For this review, take the finished solid that the model builds, in its own axes (mm). Face numbers are marked on the shaded views. Round coordinates to 2 decimals unless told otherwise and drop trailing zeros. Loops run counter-clockwise (first coordinate to the right, second up) from the corner with the lowest first, then second, coordinate; pieces in that order, holes last. Notation, with made-up numbers: M 28,-36 L 36,-36 A20 cw 36,-15 Z; hole C 12,21.5 d4. An arc over 180 degrees is marked long. Write item = value, one per line. Start each with the question number.
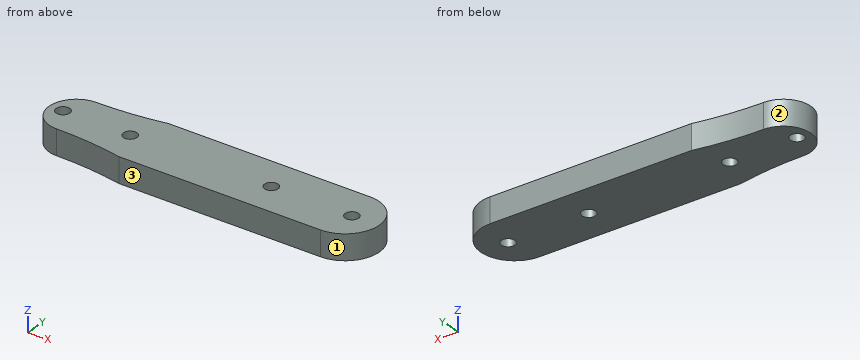
```python
from build123d import *

# Parameters (mm, degrees)
SKETCH1_R           = 1
BOSS_EXTRUDE1_DEPTH = 3.7


with BuildPart() as part:
    # Sketch1 → Boss-Extrude1 (new body)
    with BuildSketch(Plane.XY):
        with BuildLine():
            Line((0, 5), (30, 5))
            ThreePointArc((30, 5), (35, 0), (30, -5))
            Line((30, -5), (0, -5))
            ThreePointArc((0, -5), (-4.975062189, -4.250621894), (-10, -4))
            ThreePointArc((-10, -4), (-14, 0), (-10, 4))
            ThreePointArc((-10, 4), (-4.975062189, 4.250621894), (0, 5))
        make_face()
        with Locations((-12, 0)):
            Circle(SKETCH1_R, mode=Mode.SUBTRACT)
        with Locations((-2, 0)):
            Circle(SKETCH1_R, mode=Mode.SUBTRACT)
        with Locations((19, 0)):
            Circle(SKETCH1_R, mode=Mode.SUBTRACT)
        with Locations((31, 0)):
            Circle(SKETCH1_R, mode=Mode.SUBTRACT)
    extrude(amount=BOSS_EXTRUDE1_DEPTH)


solid = part.part
```
(1) Add section A-A on x = 19. Write out the cut boundary in (y, z), and give its area (3 significant figures).
(2) Draft analysis for pull direction X (two halves, no side actions). For the marked faces 1, 2 and 3, state which applies: +X half, -X half, draft (parallel to the pull), parting line (faces both ways), or undercut.
(3) For pin 1 Ø1.2 at (x, y) = (-2, 0) entering from -Z, flat-tipped, find the tip position at first contact; note if it passes through.
(4) Wall thickness on L1, parallel to X at y = 0.25, z = 1.55; L2, parallel to X at y = 0.75, z = 1.15; L3, parallel to Y at x = -12, z = 1.65: over which ranges is each line inside the solid? List them lowest first.
(5) Add section D-D on x = -2. Write out the cut boundary in (y, z), and give its area (3 significant figures).
(6) Add section C-C on y = 0. Write out the cut boundary in (x, z), and give its area (3 significant figures).
(7) Add section B-B on z = 0.5. Write out the cut boundary in (x, y), and give its area (3 significant figures).
Answer sheet:
q1.outline = M -5,0 L -1,0 L -1,3.7 L -5,3.7 Z; M 1,0 L 5,0 L 5,3.7 L 1,3.7 Z
q1.area = 29.6 mm²
q2.face_1 = +X half
q2.face_2 = -X half
q2.face_3 = draft
q3.pin_1 = through
q4.L1 = -13.99 to -12.97, -11.03 to -2.97, -1.03 to 18.03, 19.97 to 30.03, 31.97 to 34.99
q4.L2 = -13.93 to -12.66, -11.34 to -2.66, -1.34 to 18.34, 19.66 to 30.34, 31.66 to 34.94
q4.L3 = -3.46 to -1, 1 to 3.46
q5.outline = M -4.64,0 L -1,0 L -1,3.7 L -4.64,3.7 Z; M 1,0 L 4.64,0 L 4.64,3.7 L 1,3.7 Z
q5.area = 26.9 mm²
q6.outline = M -14,0 L -13,0 L -13,3.7 L -14,3.7 Z; M -11,0 L -3,0 L -3,3.7 L -11,3.7 Z; M -1,0 L 18,0 L 18,3.7 L -1,3.7 Z; M 20,0 L 30,0 L 30,3.7 L 20,3.7 Z; M 32,0 L 35,0 L 35,3.7 L 32,3.7 Z
q6.area = 152 mm²
q7.outline = M -10,-4 A50.5 cw 0,-5 L 30,-5 A5 ccw 30,5 L 0,5 A50.5 cw -10,4 A4 ccw Z; hole C -12,0 d2; hole C -2,0 d2; hole C 19,0 d2; hole C 31,0 d2
q7.area = 438 mm²
